```python
from build123d import *

# Parameters (mm, degrees)
F1_DEPTH = 1282.7
F2_R     = 4.7625
F3_DEPTH = 38.101


with BuildPart() as f1:
    # F0 (on Top) → F1 (new body)
    with BuildSketch(Plane.XY):
        Polygon((0, 3.175), (0, 0), (38.1, 0), (38.1, 38.1), (34.925, 38.1), (34.925, 3.175), align=None)
    extrude(amount=F1_DEPTH)

    # F2 (on face) → F3 (cut, through all)
    with BuildSketch(Plane.XZ):
        with Locations((19.001344, 1181.1)):
            Circle(F2_R)
        with Locations((19.001344, 165.1)):
            Circle(F2_R)
    extrude(amount=-F3_DEPTH, mode=Mode.SUBTRACT)


solid = f1.part
```
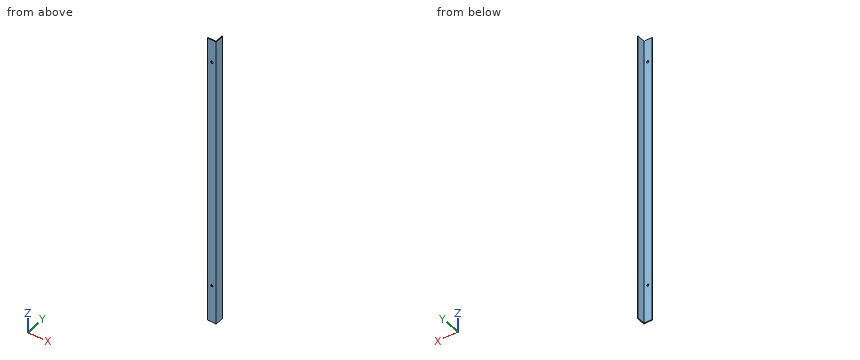
Check sheet for the modelled part. Datum: model origin and axes. Units: mm. Round coordinates to 2 decimals unless told otherwise and drop trailing zeros. Loops run counter-clockwise (first coordinate to the right, second up) from the corner with the lowest first, then second, coordinate; pieces in that order, holes last. Notation, with made-up numbers: (-32, 36) - (-3, 36) arc R18 cw to (-3, 45) - close; hole circle Ø11 at (-32, 80). An arc over 180 degrees is marked (long way). Write item = value, one per line. Start each with the question number.
Q1. Section check B-B (y = 31.5). Record the boundary of the cut face in (x, z) (3 decimals).
Q2. Thickness scan on L1, parallel to X at y = 1, z = 165; L2, parallel to Y at x = 26.5, z = 1107 (3 decimals); L3, parallel to X at y = 14.5, z = 421 (3 decimals). Record the ranges inside material, lowest first.
Q3. Section check A-A (z = 323). Record the boundary of the cut face in (x, y) (3 decimals), plus the area to 3 significant figures.
Q4. Depth check by flat-ended pin: P1, Ø6, axis at x = 14, z = 287, coming from the +Y side (3 decimals); P2, Ø2, axis at y = 8, z = 983.5, coming from the -X side (3 decimals). Enter the tip coordinate at first touch or a pass-through.
Derived:
q1.outline = (34.925, 0) - (38.1, 0) - (38.1, 1282.7) - (34.925, 1282.7) - close
q2.L1 = 0 to 14.24, 23.76 to 38.1
q2.L2 = 0 to 3.175
q2.L3 = 34.925 to 38.1
q3.outline = (0, 0) - (38.1, 0) - (38.1, 38.1) - (34.925, 38.1) - (34.925, 3.175) - (0, 3.175) - close
q3.area = 232 mm^2
q4.P1 = 3.175
q4.P2 = 34.925
